Can you work these out from the model? Positions are in its coordinate system, mm. Face numbers are marked on the shaded views. A direction names the side the tool comes from. Coordinates: 2 decimals unless noted, no trailing zeros. Loops run counter-clockwise (first coordinate to the right, second up) from the corner with the lowest first, then second, coordinate; pieces in that order, holes last.
```python
from build123d import *

# Parameters (mm, degrees)
SKETCH1_W           = 20
SKETCH1_H           = 14.5
BOSS_EXTRUDE1_DEPTH = 3
SKETCH2_W           = 3.7
SKETCH2_H           = 3.5
SKETCH2_W_2         = 3.9
SKETCH2_W_3         = 5.2
CUT_EXTRUDE1_DEPTH  = 3
CUT_EXTRUDE2_DEPTH  = 3
SKETCH4_W           = 6.213336345
SKETCH4_H           = 2.9
CUT_EXTRUDE3_DEPTH  = 10


with BuildPart() as part:
    # Sketch1 → Boss-Extrude1 (new body)
    with BuildSketch(Plane.XY):
        with Locations((2.116182573, -2.915975104)):
            Rectangle(SKETCH1_W, SKETCH1_H)
    extrude(amount=BOSS_EXTRUDE1_DEPTH)

    # Sketch2 → Cut-Extrude1 (cut)
    with BuildSketch(Plane.XY.offset(3)):
        with Locations((-6.033817427, -8.415975104)):
            Rectangle(SKETCH2_W, SKETCH2_H)
        with Locations((1.366182573, -8.415975104)):
            Rectangle(SKETCH2_W_2, SKETCH2_H)
        with Locations((9.516182573, -8.415975104)):
            Rectangle(SKETCH2_W_3, SKETCH2_H)
    extrude(amount=-CUT_EXTRUDE1_DEPTH, mode=Mode.SUBTRACT)

    # Sketch3 → Cut-Extrude2 (cut)
    with BuildSketch(Plane.XY.offset(3)):
        with BuildLine():
            Line((2.377974825, 4.334024896), (2.377974825, -1.938179145))
            ThreePointArc((2.377974825, -1.938179145), (0.927974825, -3.388179145), (-0.522025175, -1.938179145))
            Line((-0.522025175, -1.938179145), (-0.522025175, 4.334024896))
            ThreePointArc((-0.522025175, 4.334024896), (0.927974825, 5.784024896), (2.377974825, 4.334024896))
        make_face()
    extrude(amount=-CUT_EXTRUDE2_DEPTH, mode=Mode.SUBTRACT)

    # Sketch4 → Cut-Extrude3 (cut)
    with BuildSketch(Plane.XY.offset(3)):
        with Locations((-2.178693348, -1.938179145)):
            Rectangle(SKETCH4_W, SKETCH4_H)
    extrude(amount=-CUT_EXTRUDE3_DEPTH, mode=Mode.SUBTRACT)


solid = part.part
```
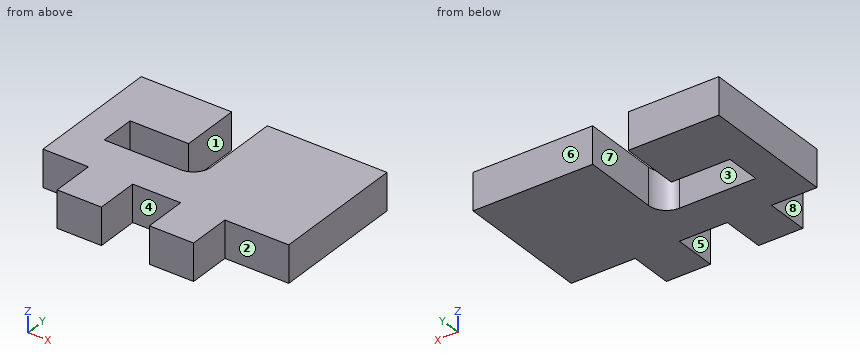
(1) If I drill on probe 1 along X at (y, z) = (2.75, 1.6); probe 2 along X at (y, z) = (-9.5, 1.3); probe 3 along Y at (x, z) = (-4.5, 2.75), over which ranges is the centre line in solid material (lowest first)?
Check values:
probe 1: x = -7.88 to -0.52, 2.38 to 12.12
probe 2: x = -4.18 to -0.58, 3.32 to 6.92
probe 3: y = -6.67 to -3.39, -0.49 to 4.33
(2) I want a section at C-C on z = 2.7. Write out the boundary of the cut face in (x, y), then the cut area to 3 significant figures.
Check values:
outline: (-7.88, -6.67) - (-4.18, -6.67) - (-4.18, -10.17) - (-0.58, -10.17) - (-0.58, -6.67) - (3.32, -6.67) - (3.32, -10.17) - (6.92, -10.17) - (6.92, -6.67) - (12.12, -6.67) - (12.12, 4.33) - (2.38, 4.33) - (2.38, -1.94) arc R1.45 cw to (0.93, -3.39) - (-5.29, -3.39) - (-5.29, -0.49) - (-0.52, -0.49) - (-0.52, 4.33) - (-7.88, 4.33) - close
area: 209 mm2
(3) I want a section at D-D on x = 7.25. Write out the boundary of the cut face in (y, z).
Check values:
outline: (-6.67, 0) - (4.33, 0) - (4.33, 3) - (-6.67, 3) - close
(4) I'm going to push flat-ended pins straight in: pin 1 (0.9 mm diameter, centred on y = -9.5, z = 2, fed in from +X); pin 2 (0.9 mm diameter, centred on y = -9, z = 2, fed in from -X). Where does each tip first touch, or does it pass through?
Check values:
pin 1: stops at x = 6.92
pin 2: stops at x = -4.18
(5) If we mould it in two halves opening along X, with no side actions, what happens to the marked faces 5, 6, 7 and 8? For each: released by +X, released by -X, zero draft, split by the parting line, or undercut.
Check values:
face 5: undercut
face 6: zero draft
face 7: undercut
face 8: released by -X
(6) Which directions (+Z, -Z, +X, -X, +Y, -Y) give clear straight access to the entire face, cutting with the end or side of a thin tool? Please do the marked faces 1, 2, 3 and 4.
Check values:
face 1: +Z, -Z, +Y
face 2: +Z, -Z, +X, -Y
face 3: +Z, -Z
face 4: +Z, -Z, -Y
(7) I want a section at A-A on x = -1.5. Write out the boundary of the cut face in (y, z), then the cut area to 3 significant figures.
Check values:
outline: (-10.17, 0) - (-3.39, 0) - (-3.39, 3) - (-10.17, 3) - close; (-0.49, 0) - (4.33, 0) - (4.33, 3) - (-0.49, 3) - close
area: 34.8 mm2
(8) I want a section at B-B on y = -1.25. Write out the boundary of the cut face in (x, z).
Check values:
outline: (-7.88, 0) - (-5.29, 0) - (-5.29, 3) - (-7.88, 3) - close; (2.38, 0) - (12.12, 0) - (12.12, 3) - (2.38, 3) - close
